Check sheet for the drawn part. Datum: minimum x, y, z corner. Units: mm. A direction names the side the tool comes from. Coordinates: 2 decimals unless noted, no trailing zeros. Write each loop counter-clockwise with the first axis right and the second up, starting at its lowest first coordinate (ties: lowest second). Pieces come first, ordered by that corner, then holes. Notation, with made-up numbers: (-3, 36.5) -> (43, 36.5) arc R27 ccw to (43, 66.5) -> close; hole circle Ø9 at (16, 68.5). An arc over 180 degrees is marked (long way). Answer in a Markdown table with one row per item. Add a question column.
Q1. Section check C-C, the plane x = 16.5. Record the boundary of the cut face in (y, z), and give its area (3 significant figures).
Q2. Section check B-B, the plane z = 9. Record the boundary of the cut face in (x, y).
Q3. Thickness scan on line 1 (Y direction, x = 39.75, z = 12.7); line 2 (Z direction, x = 37.25, y = 31.75); line 3 (X direction, y = 40, z = 13). Record the ranges inside material, lowest first.
Q4. Section check D-D, the plane y = 36. Record the boundary of the cut face in (x, z), and give its area (3 significant figures).
Q5. Tool access check on the marked faces 1, 2 and 3. Record the directions out of +Z, -Z, +X, -X, +Y, -Y that give a thin tool (end or side, any length) a straight path to the whole face; none if there is none.
Q6. Gauge pin test, flat ends, axial feed: P1, Ø10, axis at x = 73, z = 15.5, coming from the +Y side; P2, Ø10, axis at y = 27.5, z = 8, coming from the -X side; P3, Ø1.5, axis at x = 53, z = 15.5, coming from the +Y side; P4, Ø11.5, axis at y = 31.75, z = 12.7, coming from the +X side. Record the tip position at first contact, or that the pin passes through.
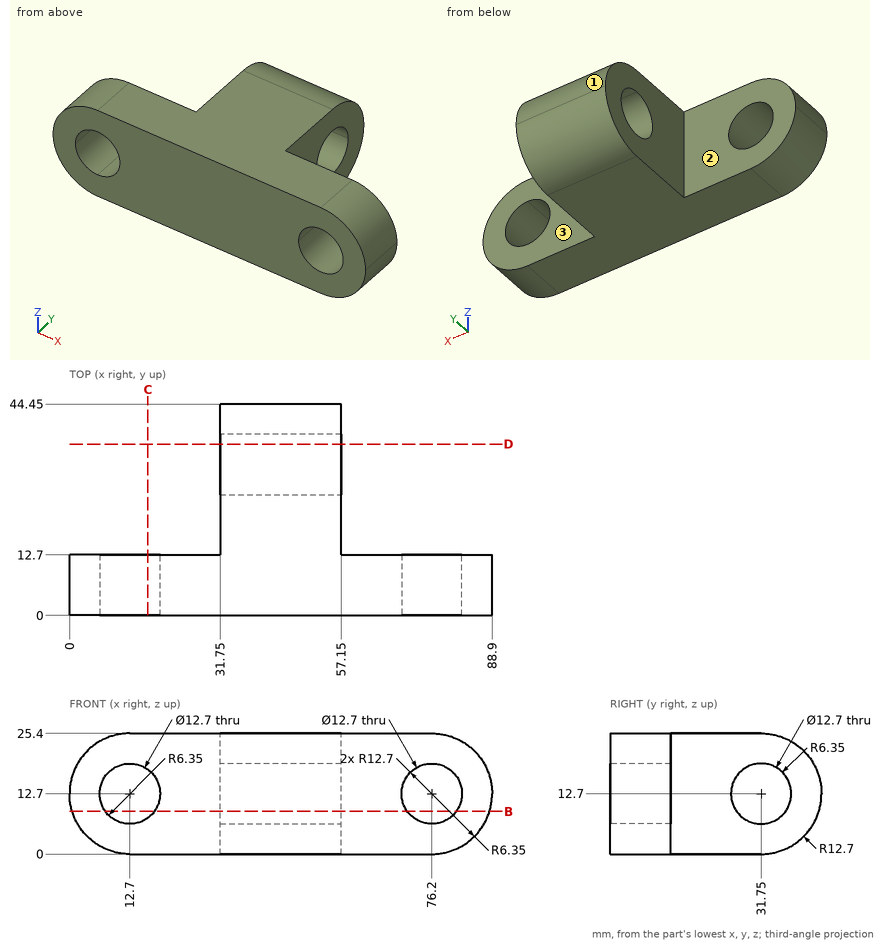
Calculated:
| question | item | result |
|---|---|---|
| 1 | outline | (0, 0) -> (12.7, 0) -> (12.7, 7.61) -> (0, 7.61) -> close; (0, 17.79) -> (12.7, 17.79) -> (12.7, 25.4) -> (0, 25.4) -> close |
| 1 | area | 193 mm² |
| 2 | outline | (0.55, 0) -> (7.54, 0) -> (7.54, 12.7) -> (0.55, 12.7) -> close; (17.86, 0) -> (71.04, 0) -> (71.04, 12.7) -> (57.15, 12.7) -> (57.15, 26.59) -> (31.75, 26.59) -> (31.75, 12.7) -> (17.86, 12.7) -> close; (31.75, 36.91) -> (57.15, 36.91) -> (57.15, 43.9) -> (31.75, 43.9) -> close; (81.36, 0) -> (88.35, 0) -> (88.35, 12.7) -> (81.36, 12.7) -> close |
| 3 | line 1 | y = 0 to 25.4, 38.1 to 44.45 |
| 3 | line 2 | z = 0 to 6.35, 19.05 to 25.4 |
| 3 | line 3 | x = 31.75 to 57.15 |
| 4 | outline | (31.75, 0.73) -> (57.15, 0.73) -> (57.15, 7.98) -> (31.75, 7.98) -> close; (31.75, 17.42) -> (57.15, 17.42) -> (57.15, 24.67) -> (31.75, 24.67) -> close |
| 4 | area | 368 mm² |
| 5 | face 1 | +Z, +X, -X, +Y |
| 5 | face 2 | +Z, -Z, -X, +Y |
| 5 | face 3 | +Z, -Z, +X, +Y |
| 6 | P1 | stops at y = 12.7 |
| 6 | P2 | stops at x = 31.75 |
| 6 | P3 | stops at y = 44.28 |
| 6 | P4 | passes through |
